from build123d import *

# Parameters (mm, degrees)
SKETCH1_W           = 20
SKETCH1_H           = 20
BOSS_EXTRUDE1_DEPTH = 6
SKETCH2_W           = 6.8
SKETCH2_H           = 20
BOSS_EXTRUDE2_DEPTH = 6
SKETCH3_W           = 7
SKETCH3_H           = 20
BOSS_EXTRUDE3_DEPTH = 15
CHAMFER1_SIZE       = 6
SKETCH4_R           = 3
CUT_EXTRUDE1_DEPTH  = 10
SKETCH5_W           = 20
SKETCH5_H           = 20
BOSS_EXTRUDE4_DEPTH = 18
CUT_EXTRUDE2_DEPTH  = 2
SKETCH7_R           = 2.8
CUT_EXTRUDE3_DEPTH  = 20
CUT_EXTRUDE4_DEPTH  = 6
SKETCH9_W           = 20
SKETCH9_H           = 8.1
BOSS_EXTRUDE5_DEPTH = 23
CUT_EXTRUDE5_REACH  = 54.058
SKETCH10_R          = 3
SKETCH11_R          = 5.05
CUT_EXTRUDE6_DEPTH  = 6.1


with BuildPart() as part:
    # Sketch1 → Boss-Extrude1 (new body)
    with BuildSketch(Plane(origin=(0, 0, 0), x_dir=(1, 0, 0), z_dir=(0, 1, 0))):
        Rectangle(SKETCH1_W, SKETCH1_H)
    extrude(amount=BOSS_EXTRUDE1_DEPTH)

    # Sketch2 → Boss-Extrude2 (add)
    with BuildSketch(Plane(origin=(0, 6, 0), x_dir=(1, 0, 0), z_dir=(0, 1, 0))):
        with Locations((6.6, 0)):
            Rectangle(SKETCH2_W, SKETCH2_H)
    extrude(amount=BOSS_EXTRUDE2_DEPTH)

    # Sketch3 → Boss-Extrude3 (add)
    with BuildSketch(Plane(origin=(0, 6, 0), x_dir=(1, 0, 0), z_dir=(0, 1, 0))):
        with Locations((-6.5, 0)):
            Rectangle(SKETCH3_W, SKETCH3_H)
    extrude(amount=BOSS_EXTRUDE3_DEPTH)

    # Chamfer1
    chamfer1_edges = [part.edges().sort_by_distance(p)[0] for p in [
        (-10, 21, 0),
    ]]
    chamfer(chamfer1_edges, length=CHAMFER1_SIZE)

    # Sketch4 → Cut-Extrude1 (cut)
    with BuildSketch(Plane(origin=(-12.5, 12.5, 0), x_dir=(0, 0, 1), z_dir=(-0.7071067811865489, 0.7071067811865462, 0))):
        with Locations(Location((0, 7.432512212, 0), (0, 0, 270))):
            Circle(SKETCH4_R)
    extrude(amount=-CUT_EXTRUDE1_DEPTH, mode=Mode.SUBTRACT)

    # Sketch5 → Boss-Extrude4 (add)
    with BuildSketch(Plane.XZ):
        Rectangle(SKETCH5_W, SKETCH5_H)
    extrude(amount=BOSS_EXTRUDE4_DEPTH)

    # Sketch6 → Cut-Extrude2 (cut)
    with BuildSketch(Plane(origin=(-12.5, 12.5, 0), x_dir=(0, 0, 1), z_dir=(-0.7071067811865489, 0.7071067811865462, 0))):
        Polygon((0, 13.8411002), (-5.55, 10.636806206), (-5.55, 4.228218218), (0, 1.023924224), (5.55, 4.228218218), (5.55, 10.636806206), align=None)
    extrude(amount=-CUT_EXTRUDE2_DEPTH, mode=Mode.SUBTRACT)

    # Sketch7 → Cut-Extrude3 (cut)
    with BuildSketch(Plane(origin=(0, -18, 0), x_dir=(-1, 0, 0), z_dir=(0, -1, 0))):
        with Locations(Location((0, 0, 0), (0, 0, 90))):
            Circle(SKETCH7_R)
    extrude(amount=-CUT_EXTRUDE3_DEPTH, mode=Mode.SUBTRACT)

    # Sketch8 → Cut-Extrude4 (cut)
    with BuildSketch(Plane(origin=(0, -18, 0), x_dir=(-1, 0, 0), z_dir=(0, -1, 0))):
        Polygon((5.088506171, -2.964305137), (5.111416639, 2.924623043), (0.022910468, 5.88892818), (-5.088506171, 2.964305137), (-5.111416639, -2.924623043), (-0.022910468, -5.88892818), align=None)
    extrude(amount=-CUT_EXTRUDE4_DEPTH, mode=Mode.SUBTRACT)

    # Sketch9 → Boss-Extrude5 (add)
    with BuildSketch(Plane(origin=(10, 0, 0), x_dir=(0, 0, -1), z_dir=(1, 0, 0))):
        with Locations((0, -13.95)):
            Rectangle(SKETCH9_W, SKETCH9_H)
    extrude(amount=BOSS_EXTRUDE5_DEPTH)

    # Sketch10 → Cut-Extrude5 (cut, up to next)
    with BuildSketch(Plane.XZ.offset(18), mode=Mode.PRIVATE) as cut_extrude5_sk1:
        with Locations(Location((25, 0, 0), (0, 0, 270))):
            Circle(SKETCH10_R)
    cut_extrude5_tool1 = extrude(cut_extrude5_sk1.sketch, amount=-CUT_EXTRUDE5_REACH, mode=Mode.PRIVATE) & part.part
    add(cut_extrude5_tool1.solids().sort_by_distance((25, -18, 0))[0], mode=Mode.SUBTRACT)

    # Sketch11 → Cut-Extrude6 (cut)
    with BuildSketch(Plane(origin=(0, -9.9, 0), x_dir=(1, 0, 0), z_dir=(0, 1, 0))):
        with Locations(Location((25, 0, 0), (0, 0, 270))):
            Circle(SKETCH11_R)
    extrude(amount=-CUT_EXTRUDE6_DEPTH, mode=Mode.SUBTRACT)


solid = part.part
Could you check a few things on this model? Use its own coordinates, in mm. A direction names the side the tool comes from. Coordinates: 2 decimals unless noted, no trailing zeros. Write each loop counter-clockwise with the first axis right and the second up, starting at its lowest first coordinate (ties: lowest second). Pieces come first, ordered by that corner, then holes. Notation, with made-up numbers: M 53.25,58 L 69.25,58 A20 ccw 69.25,78 Z; hole C 17,27.5 d6. An arc over 180 degrees is marked long. One line per question, with ' | ' between items.
1) Imagine slicing it at A-A, the plane x = 25. Write out the boundary of the cut face in (y, z).
Checks:
outline: M -18,-10 L -9.9,-10 L -9.9,-5.05 L -16,-5.05 L -16,-3 L -18,-3 Z; M -18,3 L -16,3 L -16,5.05 L -9.9,5.05 L -9.9,10 L -18,10 Z
2) For faces 5 (the face through (-7, 17, -5.55)), 6 (the face through (-3, 10, 2)), 7 (the face through (-2.603, -15.042, -4.386)), 8 (the face through (19, -9.9, 0)), which set-ups out of +Z, -Z, +X, -X, +Y, -Y let a thin tool reach every point of the face, with its end or its side?
Checks:
face 5: none | face 6: +Z, -Z, +Y | face 7: -Y | face 8: +Z, -Z, +X, +Y
3) For pin 1 Ø4.5 at (x, z) = (0.5, 0.5) entering from -Y; pin 2 Ø4 at (x, z) = (18, 8) entering from +Y; pin 3 Ø3 at (x, z) = (27, -1) entering from +Y; pin 4 Ø3.5 at (x, z) = (25, 0) entering from +Y, each with a flat end and sliding along its axis, tell me the tip position at first contact or that it passes through.
Checks:
pin 1: y = -12 | pin 2: y = -9.9 | pin 3: y = -16 | pin 4: through
4) I need wall thicknesses on probe 1 along X at (y, z) = (-3.75, 0); probe 2 along X at (y, z) = (6.5, 3.5); probe 3 along X at (y, z) = (-15, 3.5). Which ranges of each line are inside material? Lowest first, please. Write a range as [from, to].
Checks:
probe 1: [-10, -2.8], [2.8, 10] | probe 2: [-10, -3], [3.2, 10] | probe 3: [-10, -4.15], [4.12, 21.36], [28.64, 33]
5) If we mould it in two halves opening along Z, with no side actions, what happens to faces 1 (the face through (-5.963, 12.427, 0.901)), 2 (the face through (-3.72, 19.89, 4.17)), 3 (the face through (-10, -1, 0)), 4 (the face through (6, -3, -10))? For each: released by +Z, released by -Z, zero draft, split by the parting line, or undercut.
Checks:
face 1: undercut | face 2: undercut | face 3: zero draft | face 4: released by -Z
6) Imagine slicing it at B-B, the plane y = -14.5. Write out the boundary of the cut face in (x, z).
Checks:
outline: M -10,-10 L 33,-10 L 33,10 L -10,10 Z; hole M -5.11,-2.92 L -0.02,-5.89 L 5.09,-2.96 L 5.11,2.92 L 0.02,5.89 L -5.09,2.96 Z; hole C 25,0 d10.1
7) Imagine slicing it at D-D, the plane y = -5. Write out the boundary of the cut face in (x, z).
Checks:
outline: M -10,-10 L 10,-10 L 10,10 L -10,10 Z; hole C 0,0 d5.6
8) Imagine slicing it at C-C, the plane z = 0. Give the number of separate pieces and of enclosed holes in the cut face, and give its area (3 significant figures).
Checks:
separate pieces: 3 | enclosed holes: 0 | area: 538 mm²
